Job drawing, mm, ordinate dimensions from the low corner. One solid piece. Give positions to 0.01 mm unless a question says otherwise; leave off trailing zeros. Order: outer loops, then holes, each group sorted by start corner. A loop starts at its lowest first (then second) coordinate and runs counter-clockwise, first axis right, second up. Notation, with made-up numbers: M 19,-18.75 L 57,-18.75 A14 cw 57,-14.75 Z; hole C 43,71.25 d2. An arc over 180 degrees is marked long. Put each result on its own line as item: value. Start each with the question number.
1) Cut at B-B (y = 3.81). Write the cut outline in (x, z).
2) Cut at D-D (y = 42.5). Write the cut outline in (x, z), and give its area (3 significant figures).
3) Cut at A-A (y = 54.61). Write the cut outline in (x, z).
4) Drill centre lines: line 1 (Y direction, x = 54.61, z = 1.15); line 2 (X direction, y = 31, z = 2.5). Where is each one in solid material? Low to high. Write a range as [from, to].
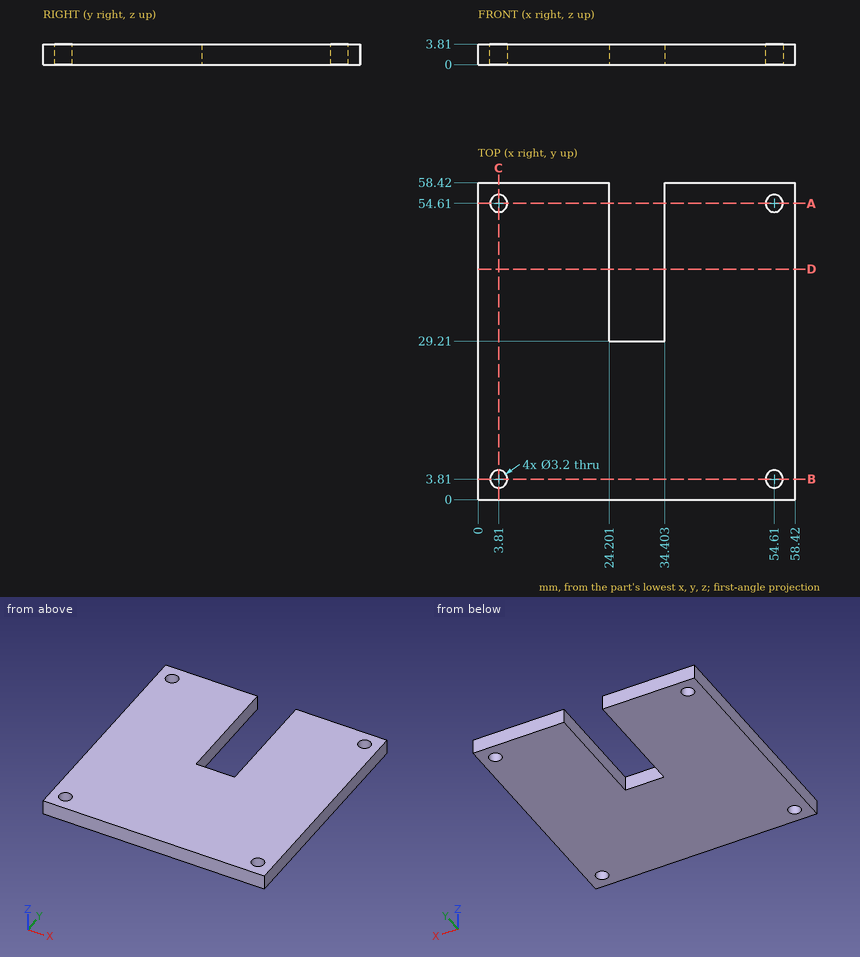
Solution:
1. outline: M 0,0 L 2.21,0 L 2.21,3.81 L 0,3.81 Z; M 5.41,0 L 53.01,0 L 53.01,3.81 L 5.41,3.81 Z; M 56.21,0 L 58.42,0 L 58.42,3.81 L 56.21,3.81 Z
2. outline: M 0,0 L 24.2,0 L 24.2,3.81 L 0,3.81 Z; M 34.4,0 L 58.42,0 L 58.42,3.81 L 34.4,3.81 Z
2. area: 184 mm²
3. outline: M 0,0 L 2.21,0 L 2.21,3.81 L 0,3.81 Z; M 5.41,0 L 24.2,0 L 24.2,3.81 L 5.41,3.81 Z; M 34.4,0 L 53.01,0 L 53.01,3.81 L 34.4,3.81 Z; M 56.21,0 L 58.42,0 L 58.42,3.81 L 56.21,3.81 Z
4. line 1: [0, 2.21], [5.41, 53.01], [56.21, 58.42]
4. line 2: [0, 24.2], [34.4, 58.42]
